Input: part model. Units: mm. Frame: model coordinates. A direction names the side the tool comes from. Round coordinates to 2 decimals unless told otherwise and drop trailing zeros. Order: outer loops, then holes, each group sorted by start corner. A loop starts at its lowest first (then second) coordinate and runs counter-clockwise, first axis right, second up. Notation, with made-up numbers: (53, -23.75) -> (61, -23.75) arc R28 ccw to (61, -0.75) -> close; hole circle Ø11 at (47.25, 17.5). An arc over 180 degrees is marked (long way). Answer as CSV lines item,"result". Start each with the question number.
1) Mould query, pull axis X, two halves, no side actions, for faces 1 (the face through (130.5, 78, 1)), 2 (the face through (120.6, 118.9, 27.4)), 3 (the face through (2, 76, -35)), 4 (the face through (-130.5, 78, 1)). Classes: +X half, -X half, draft (parallel to the pull), parting line (faces both ways), or undercut.
2) Section query A-A, the plane x = -78. Output: boundary loops of the cut face in (y, z) (3 decimals), and give its area (3 significant figures).
3) Section query B-B, the plane y = 68. Output: boundary loops of the cut face in (x, z), and give its area (3 significant figures).
4) Line query: L1, parallel to X at y = 130, z = -17; L2, parallel to X at y = 124, z = -17; L3, parallel to X at y = 103, z = 7.5. Output: solid intervals per line, ascending.
5) First-contact query: P1, Ø3, axis at x = 129, z = -4.5, coming from the +Y side (3 decimals). Flat tip, straight axial feed; report the tip coordinate or a pass-through.
6) Access query for faces 5 (the face through (-2, 132, 37.6)), 6 (the face through (111.5, 131, 27)). Directions: +Z, -Z, +X, -X, +Y, -Y. A direction counts if a zero-diameter tool reaches every point of the face in a straight line with its end or side. Return the directions, or none.
```python
from build123d import *

# Parameters (mm, degrees)
SKETCH1_W                        = 261
SKETCH1_H                        = 75.2
BOSS_EXTRUDE1_DEPTH              = 3.175
SKETCH2_W                        = 261
SKETCH2_H                        = 75.2
SKETCH2_W_2                      = 253
SKETCH2_H_2                      = 67.2
BOSS_EXTRUDE2_DEPTH              = 155
SKETCH3_W                        = 6
SKETCH3_H                        = 30
CUT_EXTRUDE1_DEPTH               = 308.496488801
SKETCH4_W                        = 9.2
SKETCH4_H                        = 20
BOSS_EXTRUDE3_DEPTH              = 15
CHAMFER2_SIZE                    = 15
F_13_0_185_DIAMETER_HOLE1_REACH  = 192.087
F_13_0_185_DIAMETER_HOLE1_BORE_R = 2.3495
LPATTERN1_COUNT                  = 3
LPATTERN1_PITCH                  = 22.4
SKETCH7_W                        = 4
SKETCH7_H                        = 15.5
SKETCH7_W_2                      = 31
SKETCH7_H_2                      = 4
CUT_EXTRUDE2_DEPTH               = 3


# Read off the part's stored shape, not the designer's step: Mirror2
with BuildPart() as part:
    # Sketch1 → Boss-Extrude1 (new body)
    with BuildSketch(Plane(origin=(0, 0, 0), x_dir=(1, 0, 0), z_dir=(0, 1, 0))):
        Rectangle(SKETCH1_W, SKETCH1_H)
    extrude(amount=BOSS_EXTRUDE1_DEPTH)

    # Sketch2 → Boss-Extrude2 (add)
    with BuildSketch(Plane(origin=(0, 3.175, 0), x_dir=(1, 0, 0), z_dir=(0, 1, 0))):
        Rectangle(SKETCH2_W, SKETCH2_H)
        Rectangle(SKETCH2_W_2, SKETCH2_H_2, mode=Mode.SUBTRACT)
    extrude(amount=BOSS_EXTRUDE2_DEPTH)

    # Sketch3 → Cut-Extrude1 (cut, through all)
    with BuildSketch(Plane(origin=(130.5, 0, 0), x_dir=(0, 0, -1), z_dir=(1, 0, 0))):
        with Locations((-34.6, 91)):
            Rectangle(SKETCH3_W, SKETCH3_H)
        with Locations((-34.6, 40)):
            Rectangle(SKETCH3_W, SKETCH3_H)
    cut_extrude1 = extrude(amount=-CUT_EXTRUDE1_DEPTH, mode=Mode.SUBTRACT)

    # Mirror1: Cut-Extrude1 across plane
    add(cut_extrude1.mirror(Plane.XY), mode=Mode.SUBTRACT)

    # Sketch4 → Boss-Extrude3 (add)
    with BuildSketch(Plane.ZY.offset(-126.5)):
        with Locations((-17.3, 123)):
            Rectangle(SKETCH4_W, SKETCH4_H)
        with Locations((27.5, 123)):
            Rectangle(SKETCH4_W, SKETCH4_H)
        with Locations((5.1, 123)):
            Rectangle(SKETCH4_W, SKETCH4_H)
    extrude(amount=BOSS_EXTRUDE3_DEPTH)

    # Chamfer2
    chamfer2_edges = [part.edges().sort_by_distance(p)[0] for p in [
        (111.5, 113, 27.5),
        (111.5, 113, 5.1),
        (111.5, 113, -17.3),
    ]]
    chamfer(chamfer2_edges, length=CHAMFER2_SIZE - 0.0001)  # a hair under: the kernel refuses the full size

    # #13 (0.185) Diameter Hole1 bore → #13 (0.185) Diameter Hole1 (cut, up to next)
    with BuildSketch(Plane(origin=(0, 133, 0), x_dir=(1, 0, 0), z_dir=(0, 1, 0)), mode=Mode.PRIVATE) as f_13_0_185_diameter_hole1_sk1:
        with Locations((117.5, -27.5)):
            Circle(F_13_0_185_DIAMETER_HOLE1_BORE_R)
    f_13_0_185_diameter_hole1_tool1 = extrude(f_13_0_185_diameter_hole1_sk1.sketch, amount=-F_13_0_185_DIAMETER_HOLE1_REACH, mode=Mode.PRIVATE) & part.part
    f_13_0_185_diameter_hole1 = f_13_0_185_diameter_hole1_tool1.solids().sort_by_distance((117.5, 133, 27.5))[0]
    add(f_13_0_185_diameter_hole1, mode=Mode.SUBTRACT)

    # LPattern1: #13 (0.185) Diameter Hole1 ×3
    with Locations(*[(0, 0, -i * LPATTERN1_PITCH) for i in range(1, LPATTERN1_COUNT)]):
        add(f_13_0_185_diameter_hole1, mode=Mode.SUBTRACT)

    # Mirror2: part across plane


with BuildPart() as part_1:
    add(part.part)
    add(part.part.mirror(Plane(origin=(0, 0, 0), x_dir=(0, 0, 1), z_dir=(1, 0, 0))))

    # Sketch7 → Cut-Extrude2 (cut)
    with BuildSketch(Plane(origin=(0, 158.175, 0), x_dir=(1, 0, 0), z_dir=(0, 1, 0))):
        with Locations((128.5, 7.75)):
            Rectangle(SKETCH7_W, SKETCH7_H)
        with Locations((48.666666667, 35.6)):
            Rectangle(SKETCH7_W_2, SKETCH7_H_2)
        with Locations((-128.5, 7.75)):
            Rectangle(SKETCH7_W, SKETCH7_H)
        with Locations((-48.666666667, 35.6)):
            Rectangle(SKETCH7_W_2, SKETCH7_H_2)
    cut_extrude2 = extrude(amount=-CUT_EXTRUDE2_DEPTH, mode=Mode.SUBTRACT)

    # Mirror3: Cut-Extrude2 across plane
    add(cut_extrude2.mirror(Plane.XY), mode=Mode.SUBTRACT)


solid = part_1.part
```
Findings:
1,face 1,"+X half"
1,face 2,"undercut"
1,face 3,"draft"
1,face 4,"-X half"
2,outline,"(0, -37.6) -> (25, -37.6) -> (25, -33.6) -> (3.175, -33.6) -> (3.175, 33.6) -> (25, 33.6) -> (25, 37.6) -> (0, 37.6) -> close; (55, -37.6) -> (76, -37.6) -> (76, -33.6) -> (55, -33.6) -> close; (55, 33.6) -> (76, 33.6) -> (76, 37.6) -> (55, 37.6) -> close; (106, -37.6) -> (158.175, -37.6) -> (158.175, -33.6) -> (106, -33.6) -> close; (106, 33.6) -> (158.175, 33.6) -> (158.175, 37.6) -> (106, 37.6) -> close"
2,area,"999 mm^2"
3,outline,"(-130.5, -37.6) -> (130.5, -37.6) -> (130.5, 37.6) -> (-130.5, 37.6) -> close; hole (-126.5, -33.6) -> (126.5, -33.6) -> (126.5, 33.6) -> (-126.5, 33.6) -> close"
3,area,"2,630 mm^2"
4,L1,"x = -130.5 to -119.83, -115.17 to -111.5, 111.5 to 115.17, 119.83 to 130.5"
4,L2,"x = -130.5 to -119.83, 119.83 to 130.5"
4,L3,"x = -130.5 to -126.5, 126.5 to 130.5"
5,P1,"stops at y = 155.175"
6,face 5,"+Z, +X, -X, +Y, -Y"
6,face 6,"+Y"
